The figure shows three views and two pictorial views of one solid part (mm, origin at its lowest corner). Answer the questions. Round coordinates to 2 decimals unless told otherwise and drop trailing zeros. Order: outer loops, then holes, each group sorted by start corner. A loop starts at its lowest first (then second) coordinate and runs counter-clockwise, first axis right, second up. Notation, with made-up numbers: M 87,-19.5 L 134,-19.5 A17 ccw 134,13.5 Z; hole C 84,45 d2. An arc over 180 degrees is marked long. Return JSON: item names as keys, results as strings.
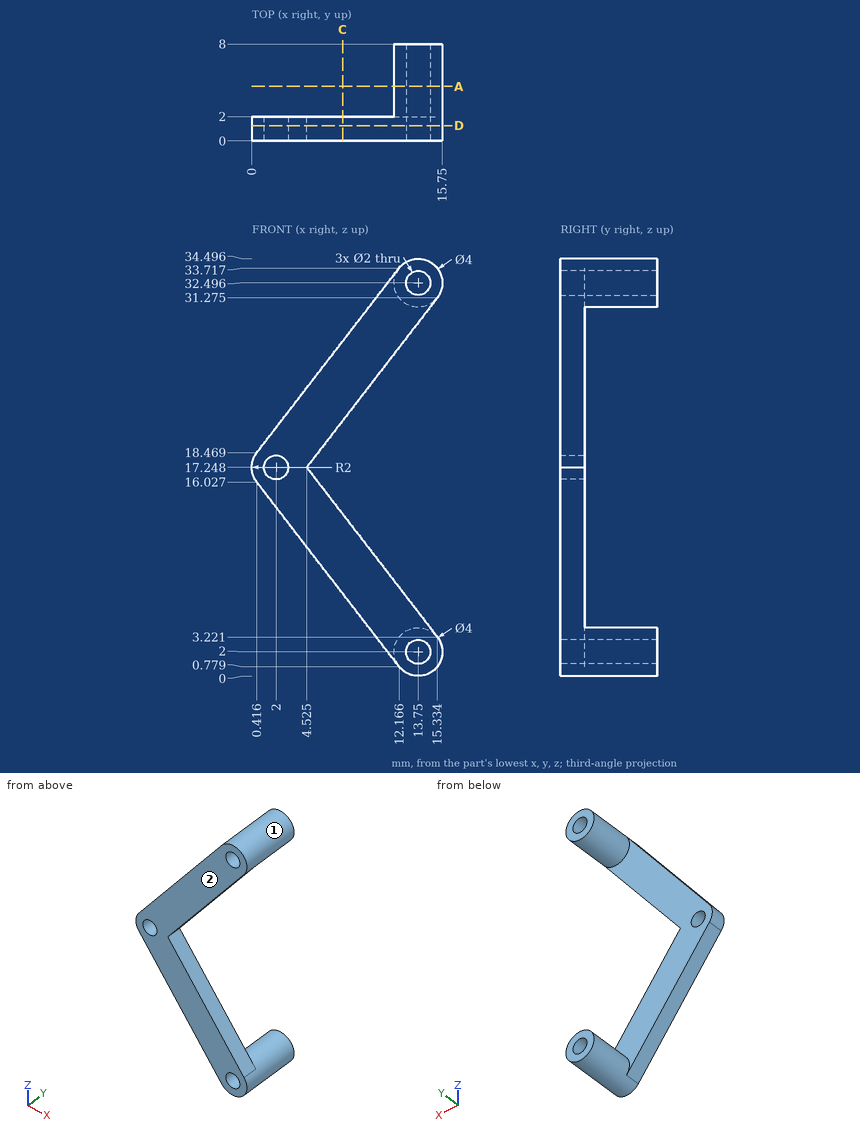
Item 1: Find section A-A (y = 4.5). Determine the outline of the cut face in (x, z).
Output:
{"outline": "C 13.75,2 d4; C 13.75,32.5 d4; hole C 13.75,2 d2; hole C 13.75,32.5 d2"}
Item 2: Consider line 1 along X through (y, z) = (4, 2); line 2 along X through (y, z) = (1, 18) (1 decimal); line 3 along Y through (x, z) = (12.75, 6). Determine where each line is inside the solid, lowest interval first. Write a range as [from, to].
Output:
{"line 1": "x = [11.75, 12.75], [14.75, 15.75]", "line 2": "x = [0.1, 1.3], [2.7, 5.1]", "line 3": "y = [0, 2]"}
Item 3: Each of these flat-tipped pins is pushed along its axis until it touches: pin 1 (1 mm diameter, centred on x = 9, z = 3.5, fed in from -Y); pin 2 (4 mm diameter, centred on x = 8.5, y = 1.5, fed in from -Z). Where does it stop, or does it pass through?
Output:
{"pin 1": "passes through", "pin 2": "stops at z = 2.94"}
Item 4: Find section C-C (x = 7.5). Determine the outline of the cut face in (y, z), plus the area to 3 significant figures.
Output:
{"outline": "M 0,6.83 L 2,6.83 L 2,13.39 L 0,13.39 Z; M 0,21.11 L 2,21.11 L 2,27.66 L 0,27.66 Z", "area": "26.2 mm^2"}
Item 5: Find section D-D (y = 1.25). State how many separate pieces and enclosed holes the cut face has, plus the area to 3 significant figures.
Output:
{"separate pieces": "1", "enclosed holes": "3", "area": "157 mm^2"}
Item 6: The mould has two halves that part along Z. Classify the marked faces 1 and 2: pulls with the +Z half, pulls with the -Z half, needs draft (parallel to the pull), parting line crosses it, or undercut.
Output:
{"face 1": "undercut", "face 2": "needs draft"}
